Autodesk Inventor part; units mm, degrees
ref_plane "Work Plane1" through (0, 0, 20) normal (0, 0, 1) x (1, 0, 0)
ref_plane "YZ Plane" through (0, 0, 0) normal (1, 0, 0) x (0, 1, 0)
ref_plane "XZ Plane" through (0, 0, 0) normal (0, 1, 0) x (-1, 0, 0)
sketch "Sketch1" plane through (0, 0, 0) normal (0, 1, 0) x (-1, 0, 0)
  circle A0 centre (0, 0) radius 20
  dimension "d0" = 40
extrude "Extrusion1" add sketch "Sketch1" along normal mid plane 100
ref_plane "Work Plane1" through (0, 0, 20) normal (0, 0, 1) x (1, 0, 0)
sketch "Sketch2" plane through (0, 0, 20) normal (0, 0, 1) x (1, 0, 0)
  line L0 (-2, -10) -> (2, -10)
  line L1 (2, -10) -> (2, -40)
  line L2 (2, -40) -> (-2, -40)
  line L3 (-2, -40) -> (-2, -10)
  point P0 (0, 0)
  dimension "d3" = 4
  dimension "d4" = 2
  dimension "d5" = 30
  dimension "d6" = 10
extrude "Extrusion2" add sketch "Sketch2" along normal blind 15 and the other way blind 5
properties part number "fuel" material "PAEK Plastic"
The listing builds one solid part. Answer for the finished solid, in the listing's coordinates (mm). A direction names the side the tool comes from. Give positions to 0.01 mm unless a question says otherwise; leave off trailing zeros. Order: outer loops, then holes, each group sorted by start corner. A loop starts at its lowest first (then second) coordinate and runs counter-clockwise, first axis right, second up.
1) Find section C-C on z = -12. Write down the section's boundary in (x, y).
Reported:
outline: (-16, -50) - (16, -50) - (16, 50) - (-16, 50) - close
2) Given P1, Ø1.2, axis at x = -1, z = 24.5, coming from the +Y side; P2, Ø1.2, axis at x = 0, z = 29, coming from the -Y side; P3, Ø7.5, axis at y = -30, z = 29, coming from the +X side, each flat-ended and moving along its own axis, determine where each tip first touches the part or whether it passes through.
Reported:
P1: stops at y = -10
P2: stops at y = -40
P3: stops at x = 2
3) Find section D-D on y = 15.5. Write down the section's boundary in (x, z).
Reported:
outline: circle Ø40 at (0, 0)
4) Find section B-B on y = -18. Write down the section's boundary in (x, z).
Reported:
outline: (-2, 19.9) arc R20 ccw (long way) to (2, 19.9) - (2, 35) - (-2, 35) - close
5) Consider line 1 along X through (y, z) = (-21, 33); line 2 along X through (y, z) = (4, 10); line 3 along Z through (x, y) = (2.5, 23.5). Determine where each line is inside the solid, lowest interval first.
Reported:
line 1: x = -2 to 2
line 2: x = -17.32 to 17.32
line 3: z = -19.84 to 19.84
6) Find section A-A on x = 0. Write down the section's boundary in (y, z), then the cut area to 3 significant figures.
Reported:
outline: (-50, -20) - (50, -20) - (50, 20) - (-10, 20) - (-10, 35) - (-40, 35) - (-40, 20) - (-50, 20) - close
area: 4,450 mm2
7) For faces 1 (the face through (0, -50, 0)), 2 (the face through (0, -10, 27)), 3 (the face through (-2, -25, 27)), 4 (the face through (2, -25, 27)), 5 (the face through (0, -40, 27)), determine the directions among +Z, -Z, +X, -X, +Y, -Y from which every point of the face is accessible in a straight line to the end or side of a thin tool.
Reported:
face 1: +Z, -Z, +X, -X, -Y
face 2: +Z, +X, -X, +Y
face 3: +Z, -X, +Y, -Y
face 4: +Z, +X, +Y, -Y
face 5: +Z, +X, -X, -Y
